from build123d import *

# Parameters (mm, degrees)
F1_DEPTH     = 25.4
F2_R         = 5.08
F3_T1_DEPTH  = 15.24
F3_T6_ANGLE  = 233.2969892374
F3_T12_ANGLE = 233.2969892374
F4_T1_DEPTH  = 31.75
F5_R         = 15.24
F6_R         = 5.08
F7_R         = 5.08
F8_R         = 5.08


# Not quite as in the source:
# - a fillet or chamfer that OpenCascade refuses, or shapes differently, is made with other operations: its cross-section is extruded or revolved along the edge and cut away or added


with BuildPart() as f1:
    # F0 (on Top) → F1 (new body)
    with BuildSketch(Plane.XY):
        Polygon((0, 6), (0, 0), (25.5269114748, 0), (38.1, 0), (76.2, 0), (76.2, 15), (74.2, 15), (74.2, 6), align=None)
        with BuildLine():
            Line((38.1, 0), (25.5269114748, 0))
            ThreePointArc((25.5269114748, 0), (43.3170296074, -12.6890998813), (38.1, -33.909))
            add(Edge.make_bspline(
                [(10.1822623983, -29.9098208), (13.5454405981, -31.48996992), (21.4109886211, -35.5910719416), (28.6130215973, -37.6913323998), (38.1, -33.909)],
                knots=[0, 0, 0, 0, 0.4439990675, 1, 1, 1, 1], degree=3))
            Line((10.1822623983, -29.9098208), (0, -29.9098208))
            Line((0, -29.9098208), (0, -34.9098208))
            Line((0, -34.9098208), (5.0913545239, -34.9098208))
            add(Edge.make_bspline(
                [(38.1, -38.909), (31.7124112149, -41.2898788749), (19.626955474, -41.5346198852), (11.6216761715, -34.9098208), (5.0913545239, -34.9098208)],
                knots=[0, 0, 0, 0, 0.512363552, 1, 1, 1, 1], degree=3))
            ThreePointArc((38.1, -38.909), (49.6761075901, -19.4545), (38.1, 0))
        make_face()
    extrude(amount=F1_DEPTH)

    # F2
    f2_edges = [f1.edges().sort_by_distance(p)[0] for p in [
        (37.1, 6, 25.4),
        (37.1, 6, 0),
    ]]
    fillet(f2_edges, radius=F2_R)

    # F3: fillet of radius 5.08 on 1 edges, made by hand

    # F3_s2 → F3_t1 (join)
    with BuildSketch(Plane.XY.offset(5.08)):
        with BuildLine():
            ThreePointArc((69.12, 6), (72.7121024484, 7.4878975516), (74.2, 11.08))
            Line((74.2, 11.08), (74.2, 6))
            Line((74.2, 6), (69.12, 6))
        make_face()
    extrude(amount=F3_T1_DEPTH)


with BuildPart() as f3_tool4:
    # F3_s5 → F3_t6 (revolve)
    with BuildSketch(Plane.XY.offset(5.08)):
        with BuildLine():
            ThreePointArc((69.12, 6), (72.7121024484, 7.4878975516), (74.2, 11.08))
            Line((74.2, 11.08), (74.2, 6))
            Line((74.2, 6), (69.12, 6))
        make_face()
    revolve(axis=Axis((74.2, 0.92, 5.08), (-1, 0, 0)), revolution_arc=F3_T6_ANGLE)

    split(bisect_by=Plane.XY, keep=Keep.TOP)

    split(bisect_by=Plane.XZ, keep=Keep.BOTTOM)


with BuildPart() as f1_1:
    add(f1.part)

    # F3_t3: union F3_tool4
    add(f3_tool4.part)


with BuildPart() as f3_tool10:
    # F3_s11 → F3_t12 (revolve)
    with BuildSketch(Plane.XY.offset(20.32)):
        with BuildLine():
            ThreePointArc((69.12, 6), (72.7121024484, 7.4878975516), (74.2, 11.08))
            Line((74.2, 11.08), (74.2, 6))
            Line((74.2, 6), (69.12, 6))
        make_face()
    revolve(axis=Axis((74.2, 0.92, 20.32), (1, 0, 0)), revolution_arc=F3_T12_ANGLE)

    split(bisect_by=Plane.XY.offset(25.4), keep=Keep.BOTTOM)

    split(bisect_by=Plane.XZ, keep=Keep.BOTTOM)


with BuildPart() as f1_2:
    add(f1_1.part)

    # F3_t9: union F3_tool10
    add(f3_tool10.part)

    # F4: fillet of radius 1.27 on 2 edges, made by hand

    # F4_s2 → F4_t1 (cut)
    with BuildSketch(Plane.XY.offset(-3.175)):
        with BuildLine():
            ThreePointArc((75.47, 15), (74.5719743879, 14.6280256121), (74.2, 13.73))
            Line((74.2, 13.73), (74.2, 15))
            Line((74.2, 15), (75.47, 15))
        make_face()
        with BuildLine():
            ThreePointArc((76.2, 13.73), (75.8280256121, 14.6280256121), (74.93, 15))
            Line((74.93, 15), (76.2, 15))
            Line((76.2, 15), (76.2, 13.73))
        make_face()
    extrude(amount=F4_T1_DEPTH, mode=Mode.SUBTRACT)

    # F5
    f5_edges = [f1_2.edges().sort_by_distance(p)[0] for p in [
        (38.1, -38.909, 12.7),
        (38.1, -33.909, 12.7),
    ]]
    fillet(f5_edges, radius=F5_R)

    # F6
    f6_edges = [f1_2.edges().sort_by_distance(p)[0] for p in [
        (38.1, 0, 12.7),
    ]]
    fillet(f6_edges, radius=F6_R)

    # F7
    f7_edges = [f1_2.edges().sort_by_distance(p)[0] for p in [
        (10.182262, -29.909821, 12.7),
    ]]
    fillet(f7_edges, radius=F7_R)

    # F8
    f8_edges = [f1_2.edges().sort_by_distance(p)[0] for p in [
        (0, 6, 12.7),
        (0, 0.46, 0),
        (0, 4.512102, 1.487898),
        (0, 4.512102, 23.912102),
        (0, 0.46, 25.4),
    ]]
    fillet(f8_edges, radius=F8_R)


solid = f1_2.part
Model file for the job. Use its own axes, mm. A direction names the side the tool comes from. Coordinates: 2 decimals unless noted, no trailing zeros. Order: outer loops, then holes, each group sorted by start corner. A loop starts at its lowest first (then second) coordinate and runs counter-clockwise, first axis right, second up. Notation, with made-up numbers: (56, 19.5) -> (97, 19.5) arc R23 ccw to (97, 38.5) -> close; hole circle Ø2 at (8.25, 13). An arc over 180 degrees is marked (long way). Return JSON: item names as keys, results as strings. Group by question number.
Item 1: Saw through at A-A on x = 48. Write the cut outline in (y, z).
Item 2: Wall check: line 1 along Z through (x, y) = (43, 1); line 2 along Y through (x, z) = (63, 5); line 3 along Y through (x, z) = (8, 12.75). Give the ranges that are in metal, low to high. Write a range as [from, to].
Item 3: Saw through at C-C on y = -17. Write the cut outline in (x, z).
Item 4: Saw through at B-B on x = 62. Write the cut outline in (y, z), then the cut area to 3 significant figures.
Item 5: Tool access for faces 1 (the flat face through (63, 0, 13)), 2 (the cylindrical face through (36.652, 4.551, 23.872)), 3 (the flat face through (38, 6, 13)), 4 (the cylindrical face through (1.449, 0.466, 1.528)): list every direction of +Z, -Z, +X, -X, +Y, -Y with a clear straight run to the whole face (end or side of a thin tool).
Item 6: Pull direction Y, two halves, no side cores. Call faces 5 (the cylindrical face through (1.449, 4.472, 12.807)), 6 (the flat face through (74.2, 12, 13)), 7 (the flat face through (3, -34.91, 13)), 8 (the flat face through (5, -29.91, 13)): pulls with the +Y half, pulls with the -Y half, needs draft (parallel to the pull), parting line crosses it, or undercut.
Item 7: Flat gauge pins, fed straight in: P1, Ø4.5, axis at x = 5.5, z = 15.5, coming from the +Y side; P2, Ø1.5, axis at x = 2.5, z = 10, coming from the -Y side; P3, Ø8, axis at y = -22, z = 18.5, coming from the -X side. Where does each tip first touch, or does it go through?
Values found:
{
 "1": {"outline": "(-27.9, 0) -> (-11.01, 0) -> (-11.01, 25.4) -> (-27.9, 25.4) -> close; (-0.75, 0) -> (0.92, 0) arc R5.08 ccw to (6, 5.08) -> (6, 20.32) arc R5.08 ccw to (0.92, 25.4) -> (-0.75, 25.4) -> close"},
 "2": {"line 1": "z = [0, 25.4]", "line 2": "y = [0, 6]", "line 3": "y = [-35.13, -29.91], [0, 6]"},
 "3": {"outline": "(44.38, 0) -> (49.54, 0) -> (49.54, 25.4) -> (44.38, 25.4) -> close"},
 "4": {"outline": "(0, 0) -> (0.92, 0) arc R5.08 ccw to (6, 5.08) -> (6, 20.32) arc R5.08 ccw to (0.92, 25.4) -> (0, 25.4) -> close", "area": "141 mm2"},
 "5": {"face 1": "+Z, -Z, +X, -Y", "face 2": "+Z, -X, +Y", "face 3": "+Z, -Z, -X, +Y", "face 4": "-Z, -X, +Y"},
 "6": {"face 5": "pulls with the +Y half", "face 6": "needs draft", "face 7": "pulls with the -Y half", "face 8": "undercut"},
 "7": {"P1": "stops at y = 6", "P2": "stops at y = -34.91", "P3": "stops at x = 43.4"}
}
